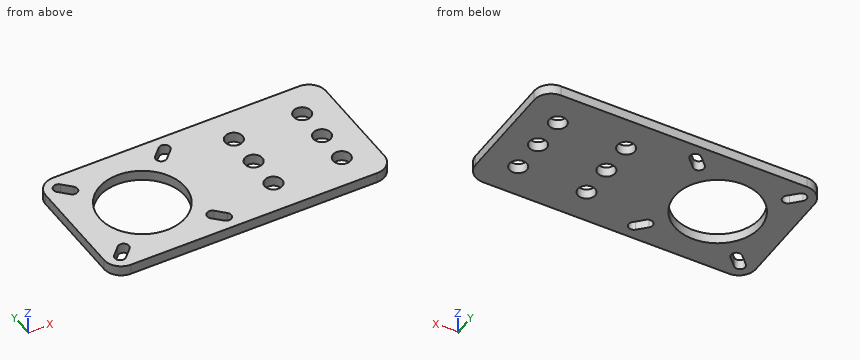
```python
from build123d import *

# Parameters (mm, degrees)
SKETCH1_W           = 82
SKETCH1_H           = 39.5
SKETCH1_R           = 12.5
SKETCH1_R_2         = 2.55
BOSS_EXTRUDE1_DEPTH = 3
FILLET1_R           = 5


with BuildPart() as part:
    # Sketch1 → Boss-Extrude1 (new body)
    with BuildSketch(Plane.XY):
        with Locations((41, 19.75)):
            Rectangle(SKETCH1_W, SKETCH1_H)
        with Locations((19.75, 19.75)):
            Circle(SKETCH1_R, mode=Mode.SUBTRACT)
        with Locations((52.3, 19.75)):
            Circle(SKETCH1_R_2, mode=Mode.SUBTRACT)
        with Locations((52.3, 29.75)):
            Circle(SKETCH1_R_2, mode=Mode.SUBTRACT)
        with Locations((52.3, 9.75)):
            Circle(SKETCH1_R_2, mode=Mode.SUBTRACT)
        with Locations((72.3, 9.75)):
            Circle(SKETCH1_R_2, mode=Mode.SUBTRACT)
        with Locations((72.3, 19.75)):
            Circle(SKETCH1_R_2, mode=Mode.SUBTRACT)
        with Locations((72.3, 29.75)):
            Circle(SKETCH1_R_2, mode=Mode.SUBTRACT)
        with BuildLine():
            Line((5.346015511, 36.346015511), (7.846015511, 33.846015511))
            ThreePointArc((7.846015511, 33.846015511), (7.846015511, 31.653984489), (5.653984489, 31.653984489))
            Line((5.653984489, 31.653984489), (3.153984489, 34.153984489))
            ThreePointArc((3.153984489, 34.153984489), (3.153984489, 36.346015511), (5.346015511, 36.346015511))
        make_face(mode=Mode.SUBTRACT)
        with BuildLine():
            Line((34.153984489, 36.346015511), (31.653984489, 33.846015511))
            ThreePointArc((31.653984489, 33.846015511), (31.653984489, 31.653984489), (33.846015511, 31.653984489))
            Line((33.846015511, 31.653984489), (36.346015511, 34.153984489))
            ThreePointArc((36.346015511, 34.153984489), (36.346015511, 36.346015511), (34.153984489, 36.346015511))
        make_face(mode=Mode.SUBTRACT)
        with BuildLine():
            Line((34.153984489, 3.153984489), (31.653984489, 5.653984489))
            ThreePointArc((31.653984489, 5.653984489), (31.653984489, 7.846015511), (33.846015511, 7.846015511))
            Line((33.846015511, 7.846015511), (36.346015511, 5.346015511))
            ThreePointArc((36.346015511, 5.346015511), (36.346015511, 3.153984489), (34.153984489, 3.153984489))
        make_face(mode=Mode.SUBTRACT)
        with BuildLine():
            Line((5.346015511, 3.153984489), (7.846015511, 5.653984489))
            ThreePointArc((7.846015511, 5.653984489), (7.846015511, 7.846015511), (5.653984489, 7.846015511))
            Line((5.653984489, 7.846015511), (3.153984489, 5.346015511))
            ThreePointArc((3.153984489, 5.346015511), (3.153984489, 3.153984489), (5.346015511, 3.153984489))
        make_face(mode=Mode.SUBTRACT)
    extrude(amount=BOSS_EXTRUDE1_DEPTH)

    # Fillet1
    fillet1_edges = [part.edges().sort_by_distance(p)[0] for p in [
        (0, 39.5, 1.5),
        (82, 39.5, 1.5),
        (82, 0, 1.5),
        (0, 0, 1.5),
    ]]
    fillet(fillet1_edges, radius=FILLET1_R)


solid = part.part
```
The listing builds one solid part. Answer for the finished solid, in the listing's coordinates (mm). Round coordinates to 2 decimals unless told otherwise and drop trailing zeros. Loops run counter-clockwise (first coordinate to the right, second up) from the corner with the lowest first, then second, coordinate; pieces in that order, holes last.
Q1. Given pin 1 Ø8 at (x, y) = (72.3, 9.75) entering from +Z, flat-ended and moving along its own axis, determine where the tip first touches the part or whether it passes through.
Q2. Section A-A, the plane y = 9.75 is taken. Determine the outline of the cut face in (x, z).
Q3. Section D-D, the plane x = 19.5 is taken. Determine the outline of the cut face in (y, z).
Q4. Section B-B, the plane x = 72.3 is taken. Determine the outline of the cut face in (y, z).
Q5. Section C-C, the plane z = 0.7 is taken. Count the separate pieces of the cut face and the enclosed holes in it, then the cut area to 3 significant figures.
Q6. Find the intervals of material crossed by line 1 (Y direction, x = 72.3, z = 2.2); line 2 (Y direction, x = 73.5, z = 1.2); line 3 (X direction, y = 10, z = 2.25), in increasing order.
Completed:
1. pin 1: stops at z = 3
2. outline: (0, 0) - (12.25, 0) - (12.25, 3) - (0, 3) - close; (27.25, 0) - (49.75, 0) - (49.75, 3) - (27.25, 3) - close; (54.85, 0) - (69.75, 0) - (69.75, 3) - (54.85, 3) - close; (74.85, 0) - (82, 0) - (82, 3) - (74.85, 3) - close
3. outline: (0, 0) - (7.25, 0) - (7.25, 3) - (0, 3) - close; (32.25, 0) - (39.5, 0) - (39.5, 3) - (32.25, 3) - close
4. outline: (0, 0) - (7.2, 0) - (7.2, 3) - (0, 3) - close; (12.3, 0) - (17.2, 0) - (17.2, 3) - (12.3, 3) - close; (22.3, 0) - (27.2, 0) - (27.2, 3) - (22.3, 3) - close; (32.3, 0) - (39.5, 0) - (39.5, 3) - (32.3, 3) - close
5. separate pieces: 1
5. enclosed holes: 11
5. area: 2,530 mm2
6. line 1: y = 0 to 7.2, 12.3 to 17.2, 22.3 to 27.2, 32.3 to 39.5
6. line 2: y = 0 to 7.5, 12 to 17.5, 22 to 27.5, 32 to 39.5
6. line 3: x = 0 to 11.93, 27.57 to 49.76, 54.84 to 69.76, 74.84 to 82
